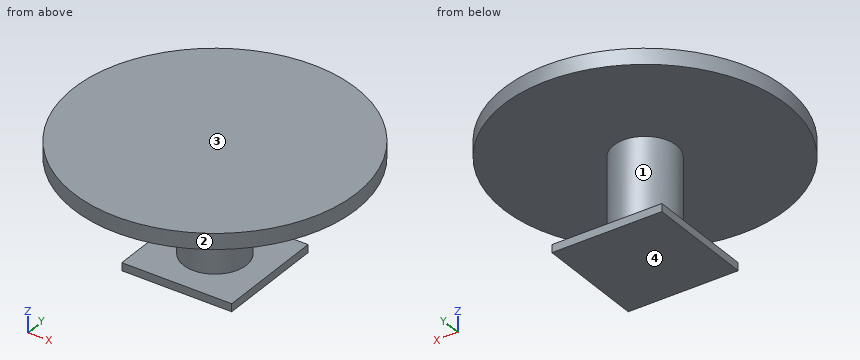
from build123d import *

# Parameters (mm, degrees)
F0_R     = 900
F0_W     = 700
F0_H     = 700
F0_R_2   = 200
F1_DEPTH = 100
F2_DEPTH = 600
F3_START = -600
F3_DEPTH = 50


with BuildPart() as f1:
    # F0 (on Top) → F1 (new body)
    with BuildSketch(Plane.XY):
        Circle(F0_R)
        Rectangle(F0_W, F0_H, mode=Mode.SUBTRACT)
        Rectangle(F0_W, F0_H)
        Circle(F0_R_2, mode=Mode.SUBTRACT)
        Circle(F0_R_2)
    extrude(amount=F1_DEPTH)

    # F0 (on Top) → F2 (join)
    with BuildSketch(Plane.XY):
        Circle(F0_R_2)
    extrude(amount=-F2_DEPTH)

    # F0 (on Top) → F3 (join)
    with BuildSketch(Plane.XY.offset(F3_START)):
        Rectangle(F0_W, F0_H)
        Circle(F0_R_2, mode=Mode.SUBTRACT)
        Circle(F0_R_2)
    extrude(amount=-F3_DEPTH)


solid = f1.part
Read the model definition and answer for the solid it produces. Units are mm, in the model's axes. Face numbers are marked on the shaded views. Coordinates: 2 decimals unless noted, no trailing zeros. Loops run counter-clockwise (first coordinate to the right, second up) from the corner with the lowest first, then second, coordinate; pieces in that order, holes last. Notation, with made-up numbers: (55, 52) - (105, 52) arc R18 cw to (105, 77) - close; hole circle Ø11 at (-18.75, 19). An arc over 180 degrees is marked (long way). Answer in a Markdown table with one row per item.
Q1. Find section C-C on x = -256. Write down the section's boundary in (y, z), plus the area to 3 significant figures.
Here are the results:
| item | result |
|---|---|
| outline | (-862.82, 0) - (862.82, 0) - (862.82, 100) - (-862.82, 100) - close; (-350, -650) - (350, -650) - (350, -600) - (-350, -600) - close |
| area | 208,000 mm^2 |
Q2. Find section D-D on y = 222. Write down the section's boundary in (x, z).
Here are the results:
| item | result |
|---|---|
| outline | (-872.19, 0) - (872.19, 0) - (872.19, 100) - (-872.19, 100) - close; (-350, -650) - (350, -650) - (350, -600) - (-350, -600) - close |
Q3. Find section A-A on x = 0. Write down the section's boundary in (y, z).
Here are the results:
| item | result |
|---|---|
| outline | (-900, 0) - (-200, 0) - (-200, -600) - (-350, -600) - (-350, -650) - (350, -650) - (350, -600) - (200, -600) - (200, 0) - (900, 0) - (900, 100) - (-900, 100) - close |
Q4. Given P1, Ø6, axis at y = 163.5, z = -155.5, coming from the -X side; P2, Ø15, axis at x = 148.5, z = -631, coming from the -Y side; P3, Ø15, axis at y = -71, z = -629.5, coming from the -X side, each flat-ended and moving along its own axis, determine where each tip first touches the part or whether it passes through.
Here are the results:
| item | result |
|---|---|
| P1 | stops at x = -119.33 |
| P2 | stops at y = -350 |
| P3 | stops at x = -350 |
Q5. Straight lines are drawn through the part: line 1 along Z through (x, y) = (171, 173.5); line 2 along Z through (x, y) = (210, -757); line 3 along X through (y, z) = (13.5, -423). For each, find the intervals that lie inside material, in ascending order. Write a range as [from, to].
Here are the results:
| item | result |
|---|---|
| line 1 | z = [-650, -600], [0, 100] |
| line 2 | z = [0, 100] |
| line 3 | x = [-199.54, 199.54] |
Q6. The mould has two halves that part along Z. Classify the marked faces 1, 2, 3 and 4: pulls with the +Z half, pulls with the -Z half, needs draft (parallel to the pull), parting line crosses it, or undercut.
Here are the results:
| item | result |
|---|---|
| face 1 | undercut |
| face 2 | needs draft |
| face 3 | pulls with the +Z half |
| face 4 | pulls with the -Z half |
